from build123d import *

# Parameters (mm, degrees)
ESQUISSE1_W        = 167
ESQUISSE1_H        = 17
BOSS_EXTRU_1_DEPTH = 3
SKETCH1_R          = 1.6
CUT_EXTRUDE1_DEPTH = 102.899460254
SKETCH2_R          = 1.6
CUT_EXTRUDE2_DEPTH = 102.899460254
SKETCH3_R          = 1.6
CUT_EXTRUDE3_DEPTH = 102.899460254


with BuildPart() as part:
    # Esquisse1 → Boss.-Extru.1 (new body)
    with BuildSketch(Plane.XY):
        with Locations((18, 0)):
            Rectangle(ESQUISSE1_W, ESQUISSE1_H)
    extrude(amount=BOSS_EXTRU_1_DEPTH)

    # Sketch1 → Cut-Extrude1 (cut, through all)
    with BuildSketch(Plane.XY.offset(3)):
        with Locations((-61.5, 2.5)):
            Circle(SKETCH1_R)
    extrude(amount=-CUT_EXTRUDE1_DEPTH, mode=Mode.SUBTRACT)

    # Sketch2 → Cut-Extrude2 (cut, through all)
    with BuildSketch(Plane(origin=(0, 0, 0), x_dir=(-1, 0, 0), z_dir=(0, 0, -1))):
        with Locations((-75.5, -4.5)):
            Circle(SKETCH2_R)
    extrude(amount=-CUT_EXTRUDE2_DEPTH, mode=Mode.SUBTRACT)

    # Sketch3 → Cut-Extrude3 (cut, through all)
    with BuildSketch(Plane.XY.offset(3)):
        with Locations((-10.5, -1.5)):
            Circle(SKETCH3_R)
    extrude(amount=-CUT_EXTRUDE3_DEPTH, mode=Mode.SUBTRACT)


solid = part.part
Model file for the job. Use its own axes, mm. Coordinates: 2 decimals unless noted, no trailing zeros. Loops run counter-clockwise (first coordinate to the right, second up) from the corner with the lowest first, then second, coordinate; pieces in that order, holes last. Notation, with made-up numbers: (-34, -25.5) -> (-2, -25.5) arc R24 ccw to (-2, -9.5) -> close; hole circle Ø4 at (85, 19). An arc over 180 degrees is marked (long way). Use one line per item in the form item = value. Start each with the question number.
(1) Probe probe 1 along Y at (x, z) = (-10.5, 1.45); probe 2 along X at (y, z) = (3, 2.8); probe 3 along X at (y, z) = (-5.5, 1.55). List the from-to ranges inside material, lowest first. Write a range as from..to.
(2) Pull direction Y, two halves, no side cores. Call faces 1 (the flat face through (17, 8.5, 1)), 2 (the flat face through (101.5, 0, 1)), 3 (the cylindrical face through (-12.1, -1.43, 1.52)): pulls with the +Y half, pulls with the -Y half, needs draft (parallel to the pull), parting line crosses it, or undercut.
(3) Cut at A-A on y = -1.5. Give the cut face in (x, z), and give its area (3 significant figures).
(4) Cut at B-B on x = 75.5. Give the cut face in (y, z).
Values:
q1.probe_1 = -8.5..-3.1, 0.1..8.5
q1.probe_2 = -65.5..-63.02, -59.98..101.5
q1.probe_3 = -65.5..74.25, 76.75..101.5
q2.face_1 = pulls with the +Y half
q2.face_2 = needs draft
q2.face_3 = undercut
q3.outline = (-65.5, 0) -> (-12.1, 0) -> (-12.1, 3) -> (-65.5, 3) -> close; (-8.9, 0) -> (101.5, 0) -> (101.5, 3) -> (-8.9, 3) -> close
q3.area = 491 mm2
q4.outline = (-8.5, 0) -> (-6.1, 0) -> (-6.1, 3) -> (-8.5, 3) -> close; (-2.9, 0) -> (8.5, 0) -> (8.5, 3) -> (-2.9, 3) -> close
